Design review of the part built by this model. Coordinates are the model's own, in mm. Face numbers are marked on the shaded views. A direction names the side the tool comes from. Round coordinates to 2 decimals unless told otherwise and drop trailing zeros. Order: outer loops, then holes, each group sorted by start corner. A loop starts at its lowest first (then second) coordinate and runs counter-clockwise, first axis right, second up. Notation, with made-up numbers: M 27.25,59 L 83.25,59 A21 cw 83.25,89 Z; hole C 26.5,32 d10. An arc over 180 degrees is marked long. Use a Markdown table: item, result. Add a question column.
(1) Machinability: for the marked faces 1, 2 and 3, which of the approach directions +Z, -Z, +X, -X, +Y, -Y give a long, thin tool a straight path to every point of the face, cutting with its end or side? Answer none if there is none.
(2) Take a section at D-D (z = -48.5). Write out the cut boundary in (x, y).
(3) For pin 1 (3 mm diameter, centred on x = 7.5, z = -33.5, fed in from -Y); pin 2 (3 mm diameter, centred on x = 18.33, z = -48.5, fed in from +Y); pin 3 (2 mm diameter, centred on y = -25, z = -39.5, fed in from +X); pin 4 (2.5 mm diameter, centred on x = 6.5, y = -6.5, fed in from +Z), all flat-tipped, find the tip position at first contact; note any pin that passes through.
(4) The part is to be moulded in two halves that separate along Z. For the marked faces 4, 5, 6 and 7, say which applies: released by +Z, released by -Z, zero draft, split by the parting line, or undercut.
(5) Take a section at C-C (y = -23). Write out the cut boundary in (x, z), then the cut area to 3 significant figures.
(6) Take a section at B-B (z = -26.5). Write out the cut boundary in (x, y), then the cut area to 3 significant figures.
(7) To check wall thickness, follow probe 1 along Z at (x, y) = (26.5, -10); probe 2 along Z at (x, y) = (17, -17.5); probe 3 along Y at (x, z) = (37, -38.5). State the ranges of each line that lie inside material, in increasing order. Write a range as from..to.
(8) Take a section at A-A (z = -10). Write out the cut boundary in (x, y).
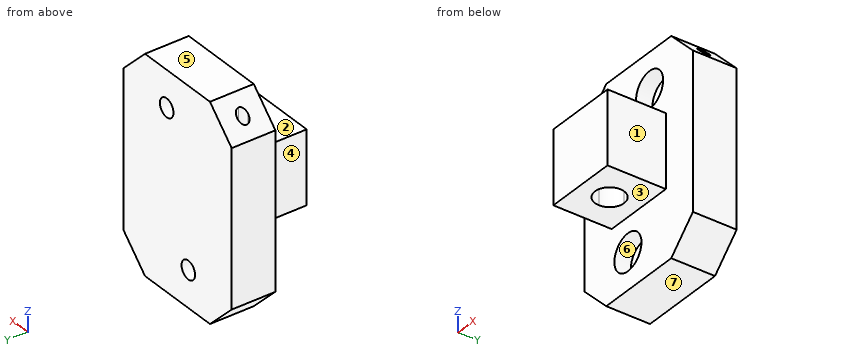
```python
from build123d import *

# Parameters (mm, degrees)
F0_R      = 2.5
F1_DEPTH  = 12
F0_W      = 10
F0_H      = 10
F2_DEPTH  = 28
F4_DEPTH  = 25
F6_DEPTH  = 16
F8_DEPTH  = 25
F10_DEPTH = 16
F11_DEPTH = 25
F13_DEPTH = 25
F14_DEPTH = 25
F16_DEPTH = 25
F18_DEPTH = 25
F19_R     = 5
F19_R_2   = 2.5
F20_DEPTH = 4.5
F21_DEPTH = 4.5


with BuildPart() as f1:
    # F0 (on Front) → F1 (new body)
    with BuildSketch(Plane.XZ):
        Polygon((22.3333325194, 0), (10.3333325194, 0), (2.3333325194, -8), (2.3333325194, -29.25), (12.3333325194, -29.25), (12.3333325194, -19.25), (22.3333325194, -19.25), align=None)
        Polygon((34.3333325194, 0), (22.3333325194, 0), (22.3333325194, -19.25), (32.3333325194, -19.25), (32.3333325194, -29.25), (42.3333325194, -29.25), (42.3333325194, -8), align=None)
        with Locations((26.3333325194, -10)):
            Circle(F0_R, mode=Mode.SUBTRACT)
        Polygon((12.3333325194, -29.25), (2.3333325194, -29.25), (2.3333325194, -50.5), (10.3333325194, -58.5), (22.3333325194, -58.5), (22.3333325194, -39.25), (12.3333325194, -39.25), align=None)
        with Locations((18.3333325194, -48.5)):
            Circle(F0_R, mode=Mode.SUBTRACT)
        Polygon((32.3333325194, -39.25), (22.3333325194, -39.25), (22.3333325194, -58.5), (34.3333325194, -58.5), (42.3333325194, -50.5), (42.3333325194, -29.25), (32.3333325194, -29.25), align=None)
    extrude(amount=F1_DEPTH)

    # F0 (on Front) → F2 (join)
    with BuildSketch(Plane.XZ):
        with Locations((17.3333325194, -24.25)):
            Rectangle(F0_W, F0_H)
        with Locations((27.3333325194, -24.25)):
            Rectangle(F0_W, F0_H)
        with Locations((27.3333325194, -34.25)):
            Rectangle(F0_W, F0_H)
        with Locations((17.3333325194, -34.25)):
            Rectangle(F0_W, F0_H)
    extrude(amount=F2_DEPTH)

    # F3 (on face) → F4 (cut)
    with BuildSketch(Plane(origin=(0, 0, 0), x_dir=(-1, 0, 0), z_dir=(0, 1, 0))):
        Polygon((-34.3333325194, 0), (-42.3333325194, -8), (-34.3333325194, -8), align=None)
    extrude(amount=-F4_DEPTH, mode=Mode.SUBTRACT)

    # F5 (on face) → F6 (cut)
    with BuildSketch(Plane.XY.offset(-8)):
        with BuildLine():
            Line((36.8333325194, -6), (38.3333325194, -6))
            Line((38.3333325194, -6), (38.3333325194, -4.5))
            ThreePointArc((38.3333325194, -4.5), (37.2726723477, -4.9393398282), (36.8333325194, -6))
        make_face()
        with BuildLine():
            Line((38.3333325194, -7.5), (38.3333325194, -6))
            Line((38.3333325194, -6), (36.8333325194, -6))
            ThreePointArc((36.8333325194, -6), (37.2726723477, -7.0606601718), (38.3333325194, -7.5))
        make_face()
        with BuildLine():
            ThreePointArc((38.3333325194, -7.5), (39.3939926912, -7.0606601718), (39.8333325194, -6))
            Line((39.8333325194, -6), (38.3333325194, -6))
            Line((38.3333325194, -6), (38.3333325194, -7.5))
        make_face()
        with BuildLine():
            Line((38.3333325194, -6), (39.8333325194, -6))
            ThreePointArc((39.8333325194, -6), (39.3939926912, -4.9393398282), (38.3333325194, -4.5))
            Line((38.3333325194, -4.5), (38.3333325194, -6))
        make_face()
    extrude(amount=-F6_DEPTH, mode=Mode.SUBTRACT)

    # F7 (on face) → F8 (cut)
    with BuildSketch(Plane(origin=(0, 0, 0), x_dir=(-1, 0, 0), z_dir=(0, 1, 0))):
        Polygon((-10.3333325194, -8), (-6.3333325194, -8), (-6.3333325194, -4), (-10.3333325194, 0), align=None)
        Polygon((-6.3333325194, -4), (-6.3333325194, -8), (-2.3333325194, -8), align=None)
    extrude(amount=-F8_DEPTH, mode=Mode.SUBTRACT)

    # F9 (on face) → F10 (cut)
    with BuildSketch(Plane.XY.offset(-8)):
        with BuildLine():
            Line((6.3333325194, -7.5), (6.3333325194, -6))
            Line((6.3333325194, -6), (4.8333325194, -6))
            ThreePointArc((4.8333325194, -6), (5.2726723477, -7.0606601718), (6.3333325194, -7.5))
        make_face()
        with BuildLine():
            Line((4.8333325194, -6), (6.3333325194, -6))
            Line((6.3333325194, -6), (6.3333325194, -4.5))
            ThreePointArc((6.3333325194, -4.5), (5.2726723477, -4.9393398282), (4.8333325194, -6))
        make_face()
        with BuildLine():
            Line((6.3333325194, -6), (7.8333325194, -6))
            ThreePointArc((7.8333325194, -6), (7.3939926912, -4.9393398282), (6.3333325194, -4.5))
            Line((6.3333325194, -4.5), (6.3333325194, -6))
        make_face()
        with BuildLine():
            ThreePointArc((6.3333325194, -7.5), (7.3939926912, -7.0606601718), (7.8333325194, -6))
            Line((7.8333325194, -6), (6.3333325194, -6))
            Line((6.3333325194, -6), (6.3333325194, -7.5))
        make_face()
    extrude(amount=-F10_DEPTH, mode=Mode.SUBTRACT)

    # F11 (add): a face of the model
    f11_faces = [f1.faces().sort_by_distance(p)[0] for p in [
        (6.3333325194, -0.144222051, -8),
    ]]
    extrude(f11_faces, amount=F11_DEPTH)

    # F12 (on face) → F13 (cut)
    with BuildSketch(Plane.XZ.offset(12)):
        Polygon((2.3333325194, -8), (10.3333325194, 0), (10.3333325194, 17), (2.3333325194, 17), align=None)
    extrude(amount=-F13_DEPTH, mode=Mode.SUBTRACT)

    # F14 (add): a face of the model
    f14_faces = [f1.faces().sort_by_distance(p)[0] for p in [
        (38.3333325194, -0.144222051, -8),
    ]]
    extrude(f14_faces, amount=F14_DEPTH)

    # F15 (on face) → F16 (cut)
    with BuildSketch(Plane.XZ.offset(12)):
        Polygon((34.3333325194, 17), (34.3333325194, 0), (42.3333325194, -8), (42.3333325194, 17), align=None)
    extrude(amount=-F16_DEPTH, mode=Mode.SUBTRACT)

    # F17 (on face) → F18 (cut)
    with BuildSketch(Plane.XY.offset(-19.25)):
        with BuildLine():
            Line((22.3333325194, -24), (22.3333325194, -20))
            Line((22.3333325194, -20), (18.3333325194, -20))
            ThreePointArc((18.3333325194, -20), (19.5049053947, -22.8284271247), (22.3333325194, -24))
        make_face()
        with BuildLine():
            Line((18.3333325194, -20), (22.3333325194, -20))
            Line((22.3333325194, -20), (22.3333325194, -16))
            ThreePointArc((22.3333325194, -16), (19.5049053947, -17.1715728753), (18.3333325194, -20))
        make_face()
        with BuildLine():
            Line((22.3333325194, -20), (26.3333325194, -20))
            ThreePointArc((26.3333325194, -20), (25.1617596442, -17.1715728753), (22.3333325194, -16))
            Line((22.3333325194, -16), (22.3333325194, -20))
        make_face()
        with BuildLine():
            ThreePointArc((22.3333325194, -24), (25.1617596442, -22.8284271247), (26.3333325194, -20))
            Line((26.3333325194, -20), (22.3333325194, -20))
            Line((22.3333325194, -20), (22.3333325194, -24))
        make_face()
    extrude(amount=-F18_DEPTH, mode=Mode.SUBTRACT)

    # F19 (on face) → F20 (cut)
    with BuildSketch(Plane.XZ.offset(12)):
        with Locations((26.3333325194, -10)):
            Circle(F19_R)
        with Locations((26.3333325194, -10)):
            Circle(F19_R_2, mode=Mode.SUBTRACT)
    extrude(amount=-F20_DEPTH, mode=Mode.SUBTRACT)

    # F19 (on face) → F21 (cut)
    with BuildSketch(Plane.XZ.offset(12)):
        with Locations((18.3333325194, -48.5)):
            Circle(F19_R)
        with Locations((18.3333325194, -48.5)):
            Circle(F19_R_2, mode=Mode.SUBTRACT)
    extrude(amount=-F21_DEPTH, mode=Mode.SUBTRACT)


solid = f1.part
```
Verdict:
| question | item | result |
|---|---|---|
| 1 | face 1 | +Z, -Z, +X, -Y |
| 1 | face 2 | +Z, +X, -X, -Y |
| 1 | face 3 | -Z, +X, -X, -Y |
| 2 | outline | M 2.33,-12 L 13.33,-12 L 13.33,-7.5 L 15.83,-7.5 L 15.83,0 L 2.33,0 Z; M 20.83,-7.5 L 23.33,-7.5 L 23.33,-12 L 42.33,-12 L 42.33,0 L 20.83,0 Z |
| 3 | pin 1 | stops at y = -12 |
| 3 | pin 2 | passes through |
| 3 | pin 3 | stops at x = 32.33 |
| 3 | pin 4 | stops at z = -2.58 |
| 4 | face 4 | zero draft |
| 4 | face 5 | released by +Z |
| 4 | face 6 | undercut |
| 4 | face 7 | released by -Z |
| 5 | outline | M 12.33,-39.25 L 19.69,-39.25 L 19.69,-19.25 L 12.33,-19.25 Z; M 24.98,-39.25 L 32.33,-39.25 L 32.33,-19.25 L 24.98,-19.25 Z |
| 5 | area | 294 mm^2 |
| 6 | outline | M 2.33,-12 L 12.33,-12 L 12.33,-28 L 32.33,-28 L 32.33,-12 L 42.33,-12 L 42.33,0 L 2.33,0 Z; hole C 22.33,-20 d8 |
| 6 | area | 750 mm^2 |
| 7 | probe 1 | z = -58.5..-15, -5..0 |
| 7 | probe 2 | z = -39.25..-19.25 |
| 7 | probe 3 | y = -12..0 |
| 8 | outline | M 2.33,-12 L 21.33,-12 L 21.33,-7.5 L 23.83,-7.5 L 23.83,0 L 2.33,0 Z; M 28.83,-7.5 L 31.33,-7.5 L 31.33,-12 L 42.33,-12 L 42.33,0 L 28.83,0 Z; hole C 6.33,-6 d3; hole C 38.33,-6 d3 |
